Geometry check sheet. Reference: the model listing, model coordinates, mm. A direction names the side the tool comes from. Coordinates: 2 decimals unless noted, no trailing zeros. Write each loop counter-clockwise with the first axis right and the second up, starting at its lowest first coordinate (ties: lowest second). Pieces come first, ordered by that corner, then holes. Notation, with made-up numbers: (-34, 88.25) - (8, 88.25) arc R21 cw to (8, 108.25) - close; hole circle Ø10 at (61.25, -20). An arc over 180 degrees is marked (long way). Answer as a JSON object with one key per item and string values. Group by question number.
from build123d import *

# Parameters (mm, degrees)
SKETCH1_W           = 25
SKETCH1_H           = 35
SKETCH1_W_2         = 15
SKETCH1_H_2         = 25
BOSS_EXTRUDE1_DEPTH = 5
SKETCH2_W           = 14
SKETCH2_H           = 1.8
BOSS_EXTRUDE2_DEPTH = 3
SKETCH3_W           = 14
SKETCH3_H           = 1.8
BOSS_EXTRUDE3_DEPTH = 3


with BuildPart() as part:
    # Sketch1 → Boss-Extrude1 (new body)
    with BuildSketch(Plane(origin=(0, 0, 0), x_dir=(1, 0, 0), z_dir=(0, 1, 0))):
        with Locations((12.5, 17.5)):
            Rectangle(SKETCH1_W, SKETCH1_H)
        with Locations((12.5, 17.5)):
            Rectangle(SKETCH1_W_2, SKETCH1_H_2, mode=Mode.SUBTRACT)
    extrude(amount=BOSS_EXTRUDE1_DEPTH)

    # Sketch2 → Boss-Extrude2 (add)
    with BuildSketch(Plane.XY):
        with Locations((12.5, 2.6)):
            Rectangle(SKETCH2_W, SKETCH2_H)
    extrude(amount=BOSS_EXTRUDE2_DEPTH)

    # Sketch3 → Boss-Extrude3 (add)
    with BuildSketch(Plane(origin=(0, 0, -35), x_dir=(-1, 0, 0), z_dir=(0, 0, -1))):
        with Locations((-12.5, 2.5)):
            Rectangle(SKETCH3_W, SKETCH3_H)
    extrude(amount=BOSS_EXTRUDE3_DEPTH)


solid = part.part
(1) Gauge pin test, flat ends, axial feed: pin 1 (1.5 mm diameter, centred on x = 10.5, z = -36, fed in from -Y); pin 2 (2 mm diameter, centred on y = 2, z = 2, fed in from -X); pin 3 (3.5 mm diameter, centred on x = 9, z = -37, fed in from +Y). Record the tip position at first contact, or that the pin passes through.
(2) Draft check along X on faces 1 (the face through (0, 2, -17)), 2 (the face through (13, 3, -38)), 3 (the face through (12, 2, -30)). Enter one of: +X half, -X half, draft (parallel to the pull), parting line (faces both ways), or undercut.
(3) Section check A-A (y = 0.8). Record the cut outline in (x, z).
(4) Material ranges on L1, parallel to Z at x = 13.75, y = 3.55; L2, parallel to X at y = 3.9, z = -20.5; L3, parallel to Z at x = 10, y = 2.5, recorded low to high. Write a range as [from, to].
(5) Section check B-B (x = 9.25). Record the cut outline in (y, z).
(6) Section check C-C (z = -11). Record the cut outline in (x, y), and give its area (3 significant figures).
(7) Set-up check for faces 4 (the face through (13, 3.4, -36)), 5 (the face through (12, 1.7, 1)), 6 (the face through (5.5, 2, -36)): record each of +Z, -Z, +X, -X, +Y, -Y from which the full face is reachable in a straight line by a thin tool's end or side.
Conclusion:
{
 "1": {"pin 1": "stops at y = 1.6", "pin 2": "stops at x = 5.5", "pin 3": "stops at y = 3.4"},
 "2": {"face 1": "-X half", "face 2": "draft", "face 3": "undercut"},
 "3": {"outline": "(0, -35) - (25, -35) - (25, 0) - (0, 0) - close; hole (5, -30) - (20, -30) - (20, -5) - (5, -5) - close"},
 "4": {"L1": "z = [-35, -30], [-5, 0]", "L2": "x = [0, 5], [20, 25]", "L3": "z = [-38, -30], [-5, 3]"},
 "5": {"outline": "(0, -35) - (1.6, -35) - (1.6, -38) - (3.4, -38) - (3.4, -35) - (5, -35) - (5, -30) - (0, -30) - close; (0, -5) - (5, -5) - (5, 0) - (3.5, 0) - (3.5, 3) - (1.7, 3) - (1.7, 0) - (0, 0) - close"},
 "6": {"outline": "(0, 0) - (5, 0) - (5, 5) - (0, 5) - close; (20, 0) - (25, 0) - (25, 5) - (20, 5) - close", "area": "50.0 mm^2"},
 "7": {"face 4": "-Z, +X, -X, +Y", "face 5": "+Z, +X, -X, -Y", "face 6": "-Z, -X, +Y, -Y"}
}
